Could you check a few things on this model? Use its own coordinates, in mm. Face numbers are marked on the shaded views. A direction names the side the tool comes from. Give positions to 0.01 mm unless a question says otherwise; leave off trailing zeros. Write each loop counter-clockwise with the first axis right and the second up, starting at its lowest first coordinate (ties: lowest second). Pieces come first, ordered by that corner, then holes. Notation, with made-up numbers: M -1.75,74.25 L 16.25,74.25 A15 ccw 16.25,88.25 Z; hole C 10.25,-38 d7. An arc over 180 degrees is marked long. One line per item, written item: value.
```python
from build123d import *

# Parameters (mm, degrees)
SKETCH1_W           = 65
SKETCH1_H           = 25
BOSS_EXTRUDE1_DEPTH = 10
SKETCH3_R           = 2
CUT_EXTRUDE1_DEPTH  = 10
SKETCH5_R           = 4.1
CUT_EXTRUDE2_DEPTH  = 3.7
SKETCH12_R          = 3
CUT_EXTRUDE3_DEPTH  = 24.2
SKETCH13_R          = 5
CUT_EXTRUDE4_DEPTH  = 6


with BuildPart() as part:
    # Sketch1 → Boss-Extrude1 (new body)
    with BuildSketch(Plane.XY):
        with Locations((-15.021367521, 0)):
            Rectangle(SKETCH1_W, SKETCH1_H)
    extrude(amount=BOSS_EXTRUDE1_DEPTH)

    # Sketch3 → Cut-Extrude1 (cut)
    with BuildSketch(Plane(origin=(0, 0, 0), x_dir=(-1, 0, 0), z_dir=(0, 0, -1))):
        with Locations((22.021367521, -7)):
            Circle(SKETCH3_R)
        with Locations((8.021367521, -7)):
            Circle(SKETCH3_R)
        with Locations((8.021367521, 7)):
            Circle(SKETCH3_R)
        with Locations((22.021367521, 7)):
            Circle(SKETCH3_R)
    extrude(amount=-CUT_EXTRUDE1_DEPTH, mode=Mode.SUBTRACT)

    # Sketch5 → Cut-Extrude2 (cut)
    with BuildSketch(Plane(origin=(0, 0, 0), x_dir=(-1, 0, 0), z_dir=(0, 0, -1))):
        with Locations((22.021367521, -7)):
            Circle(SKETCH5_R)
        with Locations((8.021367521, -7)):
            Circle(SKETCH5_R)
        with Locations((8.021367521, 7)):
            Circle(SKETCH5_R)
        with Locations((22.021367521, 7)):
            Circle(SKETCH5_R)
    extrude(amount=-CUT_EXTRUDE2_DEPTH, mode=Mode.SUBTRACT)

    # Sketch12 → Cut-Extrude3 (cut)
    with BuildSketch(Plane.XY.offset(10)):
        with Locations((-40.021367521, 0)):
            Circle(SKETCH12_R)
        with Locations((9.978632479, 0)):
            Circle(SKETCH12_R)
    extrude(amount=-CUT_EXTRUDE3_DEPTH, mode=Mode.SUBTRACT)

    # Sketch13 → Cut-Extrude4 (cut)
    with BuildSketch(Plane.XY.offset(10)):
        with Locations((-40.021367521, 0)):
            Circle(SKETCH13_R)
        with Locations((9.978632479, 0)):
            Circle(SKETCH13_R)
    extrude(amount=-CUT_EXTRUDE4_DEPTH, mode=Mode.SUBTRACT)


solid = part.part
```
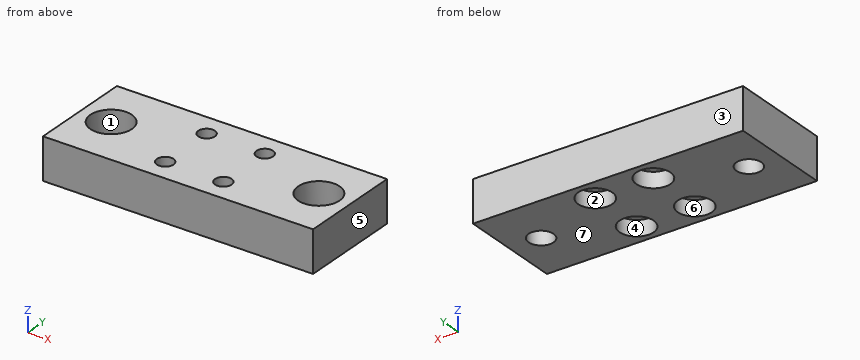
1) If we section it at C-C, the plane y = 0: Write out the boundary of the cut face in (x, z), then the cut area to 3 significant figures.
Outcome:
outline: M -47.52,0 L -43.02,0 L -43.02,4 L -45.02,4 L -45.02,10 L -47.52,10 Z; M -37.02,0 L 6.98,0 L 6.98,4 L 4.98,4 L 4.98,10 L -35.02,10 L -35.02,4 L -37.02,4 Z; M 12.98,0 L 17.48,0 L 17.48,10 L 14.98,10 L 14.98,4 L 12.98,4 Z
area: 482 mm^2
2) If we section it at A-A, the plane y = 7: Write out the boundary of the cut face in (x, z), then the cut area to 3 significant figures.
Outcome:
outline: M -47.52,0 L -26.12,0 L -26.12,3.7 L -24.02,3.7 L -24.02,10 L -47.52,10 Z; M -20.02,3.7 L -17.92,3.7 L -17.92,0 L -12.12,0 L -12.12,3.7 L -10.02,3.7 L -10.02,10 L -20.02,10 Z; M -6.02,3.7 L -3.92,3.7 L -3.92,0 L 17.48,0 L 17.48,10 L -6.02,10 Z
area: 539 mm^2
3) I'm going to push flat-ended pins straight in: pin 1 (9 mm diameter, centred on x = -20.5, y = -6.5, fed in from -Z); pin 2 (6.5 mm diameter, centred on x = -22.02, y = -7, fed in from -Z). Where does each tip first touch, or does it pass through?
Outcome:
pin 1: stops at z = 0
pin 2: stops at z = 3.7
4) We'd pull the mould along X, two halves only. Please class the marked faces 4, 5, 6 and 7: pulls with the +X half, pulls with the -X half, needs draft (parallel to the pull), parting line crosses it, or undercut.
Outcome:
face 4: undercut
face 5: pulls with the +X half
face 6: undercut
face 7: needs draft
5) If we section it at B-B, the plane z = 2.75: Write out the boundary of the cut face in (x, y), then the cut area to 3 significant figures.
Outcome:
outline: M -47.52,-12.5 L 17.48,-12.5 L 17.48,12.5 L -47.52,12.5 Z; hole C -40.02,0 d6; hole C -22.02,-7 d8.2; hole C -22.02,7 d8.2; hole C -8.02,-7 d8.2; hole C -8.02,7 d8.2; hole C 9.98,0 d6
area: 1,360 mm^2
6) If we section it at D-D, the plane x = -19: Write out the boundary of the cut face in (y, z).
Outcome:
outline: M -12.5,0 L -9.77,0 L -9.77,3.7 L -4.23,3.7 L -4.23,0 L 4.23,0 L 4.23,3.7 L 9.77,3.7 L 9.77,0 L 12.5,0 L 12.5,10 L -12.5,10 Z
7) On a 3-axis mill with a long thin cutter (end or side, diameter ignored), from which of +Z, -Z, +X, -X, +Y, -Y can I reach the whole of each face in a straight line? I mean the marked faces 1, 2 and 3. Say none if no direction works.
Outcome:
face 1: +Z
face 2: -Z
face 3: +Z, -Z, +X, -X, +Y
8) Please list where these lines run through material, in increasing order: L1, parallel to Y at x = -8, z = 9.5; L2, parallel to X at y = 4.5, z = 4.25; L3, parallel to X at y = 9.25, z = 1.5. Write a range as from..to.
Outcome:
L1: y = -12.5..-9, -5..5, 9..12.5
L2: x = -47.52..-42.2, -37.84..7.8, 12.16..17.48
L3: x = -47.52..-25.45, -18.59..-11.45, -4.59..17.48
